from build123d import *

# Parameters (mm, degrees)
SKETCH1_R           = 48
BOSS_EXTRUDE1_DEPTH = 1.5
CUT_EXTRUDE1_START  = -1.5
CUT_EXTRUDE1_DEPTH  = 1.5
CUT_EXTRUDE2_DEPTH  = 1.5


with BuildPart() as part:
    # Sketch1 → Boss-Extrude1 (new body)
    with BuildSketch(Plane(origin=(0, 0, 0), x_dir=(1, 0, 0), z_dir=(0, 1, 0))):
        with Locations(Location((0, 0, 0), (0, 0, 270))):
            Circle(SKETCH1_R)
    extrude(amount=BOSS_EXTRUDE1_DEPTH)

    # Sketch2 → Cut-Extrude1 (cut)
    with BuildSketch(Plane(origin=(0, 1.5, 0), x_dir=(1, 0, 0), z_dir=(0, 1, 0)).offset(CUT_EXTRUDE1_START)):
        with BuildLine():
            Line((-38.987177379, 28), (38.987177379, 28))
            ThreePointArc((38.987177379, 28), (0, -48), (-38.987177379, 28))
        make_face()
    extrude(amount=CUT_EXTRUDE1_DEPTH, mode=Mode.SUBTRACT)

    # Sketch3 → Cut-Extrude2 (cut)
    with BuildSketch(Plane(origin=(0, 1.5, 0), x_dir=(1, 0, 0), z_dir=(0, 1, 0))):
        Polygon((17.498096782, 40.137165991), (-14.782501595, 31.180996698), (-14.24780465, 29.253796759), (18.036697969, 38.211053647), align=None)
    extrude(amount=-CUT_EXTRUDE2_DEPTH, mode=Mode.SUBTRACT)


solid = part.part
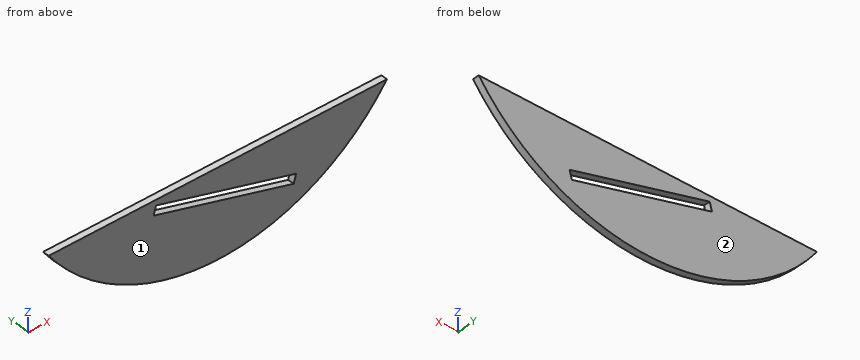
Geometry: final body of the model. Coordinates: model frame, mm. Face numbers are marked on the shaded views. Give positions to 0.01 mm unless a question says otherwise; leave off trailing zeros. Loops run counter-clockwise (first coordinate to the right, second up) from the corner with the lowest first, then second, coordinate; pieces in that order, holes last. Notation, with made-up numbers: (-7, -30) - (39, -30) arc R8 ccw to (39, -26) - close; hole circle Ø8 at (13, -32). An arc over 180 degrees is marked (long way). One line per question, with ' | ' between items. Start each with the question number.
(1) Section query C-C on y = 1.05. Return loops of the section in (x, z).
(2) Ray query, line 1 (Z direction, x = 8.5, y = 0.2); line 2 (Z direction, x = -12, y = 1.25); line 3 (X direction, y = 0.9, z = -41.75). Return the intervals inside material, ascending. Write a range as from..to.
(3) Section query B-B on x = -11.5. Return loops of the section in (y, z), then the cut area to 3 significant figures.
(4) Section query D-D on x = 27. Return loops of the section in (y, z), then the cut area to 3 significant figures.
(5) Pull-direction query (Y, two-part tool) for the marked faces 1 and 2; classes: released by +Y, released by -Y, zero draft, split by the parting line, or undercut.
(6) Section query A-A on z = -34. Return loops of the section in (x, y), then the cut area to 3 significant figures.
The answers:
1) outline: (-38.99, -28) arc R48 ccw to (38.99, -28) - close; hole (-14.78, -31.18) - (17.5, -40.14) - (18.04, -38.21) - (-14.25, -29.25) - close
2) line 1: -47.24..-37.64, -35.57..-28 | line 2: -46.48..-31.95, -29.88..-28 | line 3: -23.68..23.68
3) outline: (0, -46.6) - (1.5, -46.6) - (1.5, -32.09) - (0, -32.09) - close; (0, -30.02) - (1.5, -30.02) - (1.5, -28) - (0, -28) - close | area: 24.8 mm2
4) outline: (0, -39.69) - (1.5, -39.69) - (1.5, -28) - (0, -28) - close | area: 17.5 mm2
5) face 1: released by -Y | face 2: released by +Y
6) outline: (-33.88, 0) - (-4.62, 0) - (-4.62, 1.5) - (-33.88, 1.5) - close; (2.86, 0) - (33.88, 0) - (33.88, 1.5) - (2.86, 1.5) - close | area: 90.4 mm2
